Check sheet for the modelled part. Datum: model origin and axes. Units: mm. A direction names the side the tool comes from. Round coordinates to 2 decimals unless told otherwise and drop trailing zeros. Loops run counter-clockwise (first coordinate to the right, second up) from the corner with the lowest first, then second, coordinate; pieces in that order, holes last. Notation, with made-up numbers: (54, 5) -> (83, 5) arc R16 ccw to (83, 14) -> close; hole circle Ø4 at (66, -33.5). An arc over 180 degrees is marked (long way). Use one line per item in the form item = value. Start each with the question number.
(1) Sectioned sample at C-C (z = 1). State how many separate pieces and enclosed holes the cut face has, and give its area (3 significant figures).
(2) Go/stop test with flat-tipped pins: pin 1 (1 mm diameter, centred on x = -19, z = 7, fed in from -Y); pin 2 (24 mm diameter, centred on x = 13, y = 6.5, fed in from +Z); pin 3 (2.5 mm diameter, centred on x = -6, z = 3.5, fed in from +Y). Record where each tip stops, or that it passes through.
(3) Sectioned sample at B-B (x = 0). Record the cut outline in (y, z).
(4) Material ranges on probe 1 along Y at (x, z) = (0, 3.25); probe 2 along Y at (x, z) = (-31, 3); probe 3 along X at (y, z) = (20, 4), recorded low to high. Write a range as [from, to].
(5) Sectioned sample at A-A (y = 0). Record the cut outline in (x, z), and give its area (3 significant figures).
(6) Set-up check for faces 1 (the flat face through (32, 0, 4)), 2 (the flat face through (-18.6, 35.1, 4.1)), 3 (the flat face through (33.98, 28.74, 10.35)): record each of +Z, -Z, +X, -X, +Y, -Y from which the full face is reachable in a straight line by a thin tool's end or side.
(7) Draft check along Z on faces 4 (the flat face through (-32, 0, 4)), 5 (the flat face through (30, 34, 6)), 6 (the flat face through (33.34, -38.83, 10.03)). Enter one of: released by +Z, released by -Z, zero draft, split by the parting line, or undercut.
from build123d import *

# Parameters (mm, degrees)
SKETCH_1_W             = 80
SKETCH_1_H             = 80
EXTRUDE_1_DEPTH        = 8
SKETCH_6_R             = 13
CUT_EXTRUDE_3_DEPTH    = 50
EXTRUDE_2_DEPTH        = 12
FILLET_1_R             = 1.5
FILLET_1_OF_MIRROR_1_R = 1.5
SKETCH_8_R             = 1.3
CUT_EXTRUDE_4_DEPTH    = 10
SKETCH_9_R             = 1.3
CUT_EXTRUDE_5_DEPTH    = 10
SKETCH_10_R            = 1.6
CUT_EXTRUDE_6_DEPTH    = 10
CUT_EXTRUDE_7_DEPTH    = 10
FILLET_2_R             = 3


with BuildPart() as part:
    # 草图1 → 凸台-拉伸1 (new body)
    with BuildSketch(Plane.XY):
        Rectangle(SKETCH_1_W, SKETCH_1_H)
    extrude(amount=EXTRUDE_1_DEPTH)

    # 草图6 → 切除-拉伸3 (cut)
    with BuildSketch(Plane.XY.offset(8)):
        Circle(SKETCH_6_R)
    extrude(amount=-CUT_EXTRUDE_3_DEPTH, mode=Mode.SUBTRACT)

    # 草图7 → 凸台-拉伸2 (add)
    with BuildSketch(Plane.ZY.offset(40)):
        Polygon((8, 40), (8, 27.381197846), (12, 29.690598923), (12, 37.690598923), align=None)
        Polygon((12, -37.690598923), (8, -40), (8, -27.381197846), (12, -29.690598923), align=None)
    extrude_2 = extrude(amount=-EXTRUDE_2_DEPTH)

    # 圆角1
    fillet_1_edges = [part.edges().sort_by_distance(p)[0] for p in [
        (-28, 33.690598923, 8),
        (-34, 27.381197846, 8),
        (-28, -33.690598923, 8),
        (-34, -27.381197846, 8),
    ]]
    fillet(fillet_1_edges, radius=FILLET_1_R)

    # 镜向1: 凸台-拉伸2 across plane
    add(extrude_2.mirror(Plane(origin=(0, 0, 0), x_dir=(0, 0, 1), z_dir=(1, 0, 0))))

    # 圆角1 of 镜向1
    fillet_1_of_mirror_1_edges = [part.edges().sort_by_distance(p)[0] for p in [
        (28, 33.690598923, 8),
        (34, 27.381197846, 8),
        (28, -33.690598923, 8),
        (34, -27.381197846, 8),
    ]]
    fillet(fillet_1_of_mirror_1_edges, radius=FILLET_1_OF_MIRROR_1_R)

    # 草图8 → 切除-拉伸4 (cut)
    with BuildSketch(Plane.ZY.offset(40)):
        with Locations(Location((6, 33.690598923, 0), (0, 0, 270))):
            Circle(SKETCH_8_R)
        with Locations(Location((6, -33.690598923, 0), (0, 0, 270))):
            Circle(SKETCH_8_R)
    cut_extrude_4 = extrude(amount=-CUT_EXTRUDE_4_DEPTH, mode=Mode.SUBTRACT)

    # 镜向2: 切除-拉伸4 across plane
    add(cut_extrude_4.mirror(Plane(origin=(0, 0, 0), x_dir=(0, 0, 1), z_dir=(1, 0, 0))), mode=Mode.SUBTRACT)

    # 草图9 → 切除-拉伸5 (cut)
    with BuildSketch(Plane.XY.offset(8)):
        with Locations((7.5, -24)):
            Circle(SKETCH_9_R)
        with Locations((-7.5, -24)):
            Circle(SKETCH_9_R)
    extrude(amount=-CUT_EXTRUDE_5_DEPTH, mode=Mode.SUBTRACT)

    # 草图10 → 切除-拉伸6 (cut)
    with BuildSketch(Plane.XY.offset(8)):
        with Locations((22.5, -22.5)):
            Circle(SKETCH_10_R)
        with Locations((-22.5, -22.5)):
            Circle(SKETCH_10_R)
        with Locations((22.5, 22.5)):
            Circle(SKETCH_10_R)
        with Locations((-22.5, 22.5)):
            Circle(SKETCH_10_R)
    extrude(amount=-CUT_EXTRUDE_6_DEPTH, mode=Mode.SUBTRACT)

    # 草图11 → 切除-拉伸7 (cut)
    with BuildSketch(Plane.XY.offset(8)):
        with BuildLine():
            Line((-23.5, 40), (-14.378679656, 30.878679656))
            ThreePointArc((-14.378679656, 30.878679656), (-13.40540961, 30.228361402), (-12.257359313, 30))
            Line((-12.257359313, 30), (12.257359313, 30))
            ThreePointArc((12.257359313, 30), (13.40540961, 30.228361402), (14.378679656, 30.878679656))
            Line((14.378679656, 30.878679656), (23.5, 40))
            Line((23.5, 40), (-23.5, 40))
        make_face()
        with BuildLine():
            Line((-32, 21.178048171), (-32, -21.178048171))
            ThreePointArc((-32, -21.178048171), (-31.402395233, -22.072426909), (-30.347403579, -21.862576022))
            Line((-30.347403579, -21.862576022), (-20.28354072, -11.798713162))
            ThreePointArc((-20.28354072, -11.798713162), (-20.073689832, -11.484649115), (-20, -11.114185312))
            Line((-20, -11.114185312), (-20, 11.114185312))
            ThreePointArc((-20, 11.114185312), (-20.073689832, 11.484649115), (-20.28354072, 11.798713162))
            Line((-20.28354072, 11.798713162), (-30.347403579, 21.862576022))
            ThreePointArc((-30.347403579, 21.862576022), (-31.402395233, 22.072426909), (-32, 21.178048171))
        make_face()
        with BuildLine():
            Line((-23.5, -40), (23.5, -40))
            Line((23.5, -40), (14.378679656, -30.878679656))
            ThreePointArc((14.378679656, -30.878679656), (13.40540961, -30.228361402), (12.257359313, -30))
            Line((12.257359313, -30), (-12.257359313, -30))
            ThreePointArc((-12.257359313, -30), (-13.40540961, -30.228361402), (-14.378679656, -30.878679656))
            Line((-14.378679656, -30.878679656), (-23.5, -40))
        make_face()
        with BuildLine():
            Line((20.28354072, 11.798713162), (30.347403579, 21.862576022))
            ThreePointArc((30.347403579, 21.862576022), (31.402395233, 22.072426909), (32, 21.178048171))
            Line((32, 21.178048171), (32, -21.178048171))
            ThreePointArc((32, -21.178048171), (31.402395233, -22.072426909), (30.347403579, -21.862576022))
            Line((30.347403579, -21.862576022), (20.28354072, -11.798713162))
            ThreePointArc((20.28354072, -11.798713162), (20.073689832, -11.484649115), (20, -11.114185312))
            Line((20, -11.114185312), (20, 11.114185312))
            ThreePointArc((20, 11.114185312), (20.073689832, 11.484649115), (20.28354072, 11.798713162))
        make_face()
    extrude(amount=-CUT_EXTRUDE_7_DEPTH, mode=Mode.SUBTRACT)

    # 圆角2
    fillet_2_edges = [part.edges().sort_by_distance(p)[0] for p in [
        (-23.5, 40, 4),
        (23.5, 40, 4),
        (-23.5, -40, 4),
        (23.5, -40, 4),
    ]]
    fillet(fillet_2_edges, radius=FILLET_2_R)


solid = part.part
Checks:
q1.separate_pieces = 1
q1.enclosed_holes = 9
q1.area = 4,250 mm2
q2.pin_1 = -36
q2.pin_2 = 8
q2.pin_3 = 30
q3.outline = (-30, 0) -> (-13, 0) -> (-13, 8) -> (-30, 8) -> close; (13, 0) -> (30, 0) -> (30, 8) -> (13, 8) -> close
q4.probe_1 = [-30, -13], [13, 30]
q4.probe_2 = [-40, -22.15], [22.15, 40]
q4.probe_3 = [-40, -32], [-28.48, 28.48], [32, 40]
q5.outline = (-40, 0) -> (-32, 0) -> (-32, 8) -> (-40, 8) -> close; (-20, 0) -> (-13, 0) -> (-13, 8) -> (-20, 8) -> close; (13, 0) -> (20, 0) -> (20, 8) -> (13, 8) -> close; (32, 0) -> (40, 0) -> (40, 8) -> (32, 8) -> close
q5.area = 240 mm2
q6.face_1 = +Z, -Z
q6.face_2 = +Z, -Z, +Y
q6.face_3 = +Z, +X, -X
q7.face_4 = zero draft
q7.face_5 = undercut
q7.face_6 = released by +Z
